Job drawing, mm, ordinate dimensions from the low corner. One solid piece. Round coordinates to 2 decimals unless told otherwise and drop trailing zeros. Write each question's results on one line, items separated by ' | '. Start each with the question number.
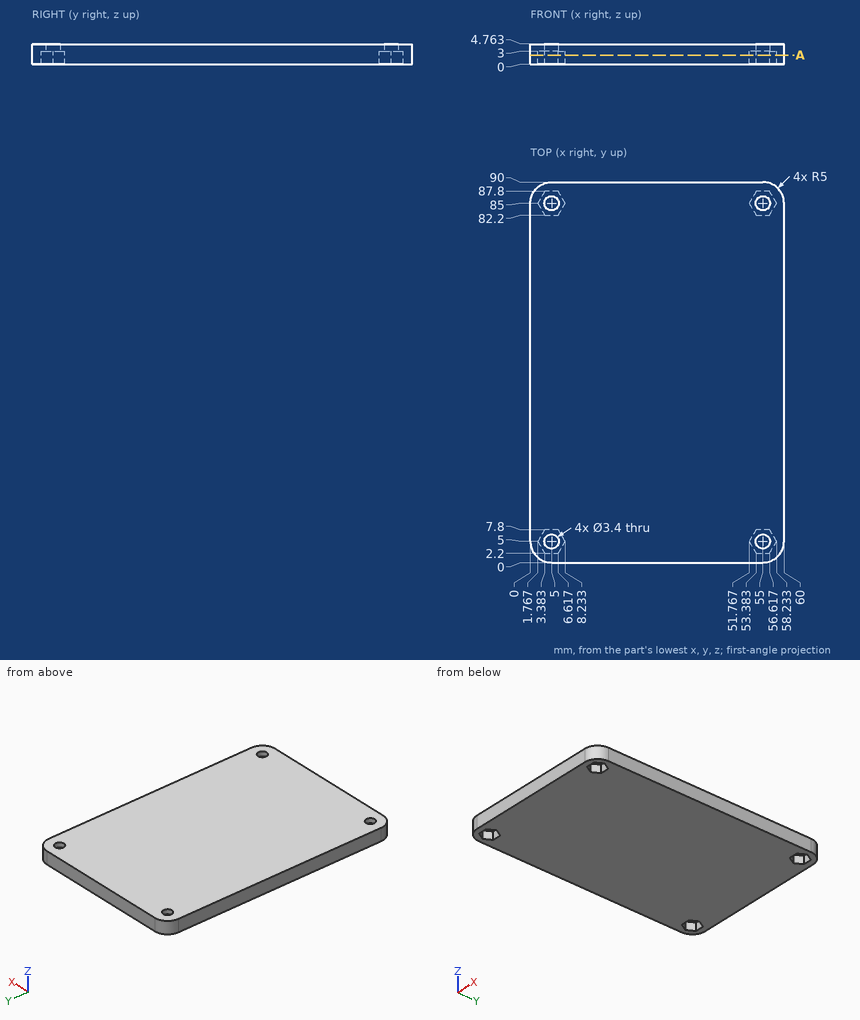
1. Flat gauge pins, fed straight in: pin 1 Ø4.5 at (x, y) = (6, 85.5) entering from -Z; pin 2 Ø4.5 at (x, y) = (54.5, 85) entering from -Z. Where does each tip first touch, or does it go through?
2. Wall check: line 1 (X direction, y = 85, z = 4.05); line 2 (Y direction, x = 55, z = 3.55); line 3 (X direction, y = 86, z = 1.25) (1 decimal). Give the ranges that are in metal, low to high. Write a range as from..to.
3. Cut at A-A (z = 2.1). Give the number of separate pieces and of enclosed holes in the cut face, plus the area to 3 significant figures.
A:
1) pin 1: stops at z = 0 | pin 2: stops at z = 3
2) line 1: x = 0..3.3, 6.7..53.3, 56.7..60 | line 2: y = 0..3.3, 6.7..83.3, 86.7..90 | line 3: x = 0.1..2.3, 7.7..52.3, 57.7..59.9
3) separate pieces: 1 | enclosed holes: 4 | area: 5,270 mm^2
